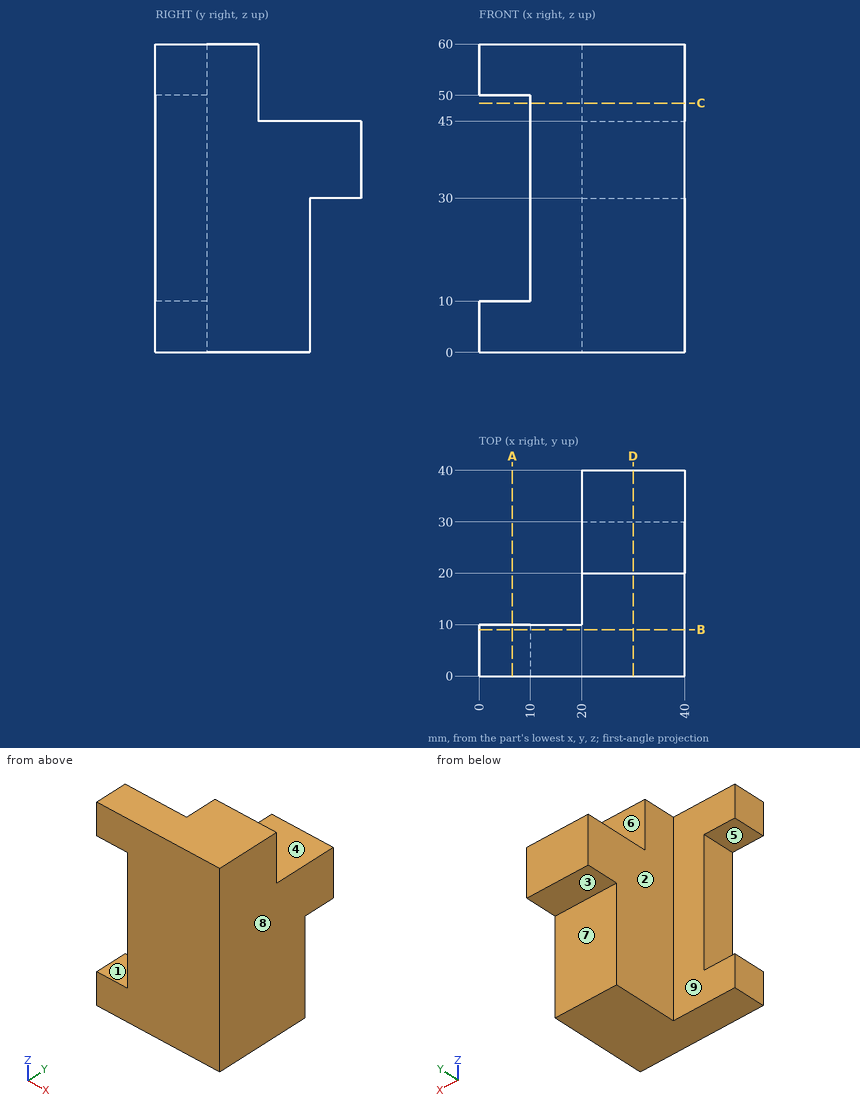
Study the drawing (mm; zero at the part's minimum x, y, z) and answer. A direction names the side the tool comes from. Give positions to 0.01 mm unless a question says otherwise; leave off trailing zeros. Write each loop counter-clockwise with the first axis right and the second up, starting at its lowest first coordinate (ties: lowest second). Pieces come first, ordered by that corner, then holes. Notation, with made-up numbers: (88, 4.25) -> (103, 4.25) arc R17 ccw to (103, 37.25) -> close; hole circle Ø3 at (50, 69). An arc over 180 degrees is marked (long way). Write item = value, one per line.
Q1. Section B-B on y = 9 is taken. Determine the outline of the cut face in (x, z).
Computed values:
outline = (0, 0) -> (40, 0) -> (40, 60) -> (0, 60) -> (0, 50) -> (10, 50) -> (10, 10) -> (0, 10) -> close
Q2. Consider line 1 along Z through (x, y) = (4.5, 5); line 2 along Z through (x, y) = (33.5, 21); line 3 along Z through (x, y) = (37, 38.5). Determine where each line is inside the solid, lowest interval first.
Computed values:
line_1 = 0 to 10, 50 to 60
line_2 = 0 to 45
line_3 = 30 to 45
Q3. For a pull along Z with two mould halves and no side action, classify the marked faces 1, 2, 3 and 4 as pulls with the +Z half, pulls with the -Z half, needs draft (parallel to the pull), parting line crosses it, or undercut.
Computed values:
face_1 = undercut
face_2 = needs draft
face_3 = pulls with the -Z half
face_4 = pulls with the +Z half
Q4. A tool of negligible diameter and unlimited length cuts with its end or side. For the marked faces 5, 6, 7, 8 and 9, from which of +Z, -Z, +X, -X, +Y, -Y can it reach the whole face along a straight path? Write none if from no direction.
Computed values:
face_5 = -X, +Y, -Y
face_6 = +Z, +X, -X, +Y
face_7 = -Z, +X, -X, +Y
face_8 = +Z, -Z, +X, +Y, -Y
face_9 = +Z, -Z, -X, +Y
Q5. Section C-C on z = 48.5 is taken. Determine the outline of the cut face in (x, y), and give its area (3 significant figures).
Computed values:
outline = (10, 0) -> (40, 0) -> (40, 20) -> (20, 20) -> (20, 10) -> (10, 10) -> close
area = 500 mm^2
Q6. Section D-D on x = 30 is taken. Determine the outline of the cut face in (y, z), and give its area (3 significant figures).
Computed values:
outline = (0, 0) -> (30, 0) -> (30, 30) -> (40, 30) -> (40, 45) -> (20, 45) -> (20, 60) -> (0, 60) -> close
area = 1,800 mm^2
Q7. Section A-A on x = 6.5 is taken. Determine the outline of the cut face in (y, z), and give its area (3 significant figures).
Computed values:
outline = (0, 0) -> (10, 0) -> (10, 10) -> (0, 10) -> close; (0, 50) -> (10, 50) -> (10, 60) -> (0, 60) -> close
area = 200 mm^2
Q8. Flat-ended cylindrical pins translate along their axes: pin 1 Ø12 at (x, y) = (25, 27) entering from +Z; pin 2 Ø16 at (x, z) = (7.5, 17.5) entering from +Y; pin 3 Ø8 at (y, z) = (3, 30.5) entering from -X. Find the tip coordinate at first contact, or state that the pin passes through.
Computed values:
pin_1 = 45
pin_2 = 10
pin_3 = 10
